from build123d import *

# Parameters (mm, degrees)
BOSS_EXTRUDE1_DEPTH      = 3
BOSS_EXTRUDE1_DEPTH_BACK = 1
CHAMFER1_SIZE            = 0.5


with BuildPart() as part:
    # Sketch2 → Boss-Extrude1 (new, two sides: drawn at the far end of the back side and taken through both)
    with BuildSketch(Plane(origin=(0, 0, 0), x_dir=(1, 0, 0), z_dir=(0, 1, 0)).offset(-BOSS_EXTRUDE1_DEPTH_BACK)):
        with BuildLine():
            Line((-9.425, 0.3), (-9.425, 0.925))
            Line((-9.425, 0.925), (-0.925, 0.925))
            Line((-0.925, 0.925), (-0.925, 9.425))
            Line((-0.925, 9.425), (0, 9.425))
            Line((0, 9.425), (0.925, 9.425))
            Line((0.925, 9.425), (0.925, 0.925))
            Line((0.925, 0.925), (9.425, 0.925))
            Line((9.425, 0.925), (9.425, 0.3))
            Line((9.425, 0.3), (11.446169588, 0.3))
            ThreePointArc((11.446169588, 0.3), (0, 11.45010036), (-11.446169588, 0.3))
            Line((-11.446169588, 0.3), (-9.425, 0.3))
        make_face()
    extrude(amount=BOSS_EXTRUDE1_DEPTH + BOSS_EXTRUDE1_DEPTH_BACK)

    # Chamfer1
    chamfer1_edges = [part.edges().sort_by_distance(p)[0] for p in [
        (-5.175, -1, -0.925),
        (-0.925, -1, -5.175),
        (0.925, 1, -0.925),
        (-0.925, 1, -0.925),
        (0.925, -1, -5.175),
        (-5.175, 3, -0.925),
        (-0.925, 3, -5.175),
        (0.925, 3, -5.175),
        (5.175, 3, -0.925),
        (5.175, -1, -0.925),
    ]]
    chamfer(chamfer1_edges, length=CHAMFER1_SIZE)


solid = part.part
Design review of the part built by this model. Coordinates are the model's own, in mm. A direction names the side the tool comes from. Coordinates: 2 decimals unless noted, no trailing zeros. Order: outer loops, then holes, each group sorted by start corner. A loop starts at its lowest first (then second) coordinate and runs counter-clockwise, first axis right, second up.
Item 1: The part is to be moulded in two halves that separate along X. For faces 1 (the cylindrical face through (0.248, 0.972, -11.447)), 2 (the flat face through (5, 1, -0.925)), 3 (the flat face through (-10, 1, -0.3)), say which applies: pulls with the +X half, pulls with the -X half, needs draft (parallel to the pull), parting line crosses it, or undercut.
Item 2: Take a section at A-A, the plane y = 1.1. Write out the cut boundary in (x, z) (3 decimals), then the cut area to 3 significant figures.
Item 3: Take a section at C-C, the plane x = 0. Write out the cut boundary in (y, z) (3 decimals).
Item 4: Take a section at B-B, the plane z = -4.75. Write out the cut boundary in (x, y) (3 decimals), then the cut area to 3 significant figures.
Item 5: Take a section at D-D, the plane z = -3.25. Write out the cut boundary in (x, y) (3 decimals).
Item 6: For line 1 (X direction, y = -0.6, z = -0.75) (3 decimals); line 2 (Z direction, x = 6.5, y = 1.8) (3 decimals); line 3 (Z direction, x = 0, y = -0.15) (3 decimals), list the stretches that pass through material, from the lowest coordinate up.
Item 7: For faces 4 (the flat face through (2, -1, -6)), 5 (the flat face through (-0.925, 1, -5)), list the 3-axis set-ups (+Z, -Z, +X, -X, +Y, -Y) from which the entire face can be reached by the end or side of a thin tool; tool diameter is ignored.
Item 8: For pin 1 Ø0.9 at (y, z) = (1, -1) entering from +X; pin 2 Ø0.6 at (y, z) = (1, -1) entering from -X; pin 3 Ø1.5 at (y, z) = (0.5, -7) entering from -X, all flat-tipped, find the tip position at first contact; note any pin that passes through.
The answers:
1. face 1: parting line crosses it
1. face 2: undercut
1. face 3: needs draft
2. outline: (-11.446, -0.3) arc R11.45 ccw to (11.446, -0.3) - (9.425, -0.3) - (9.425, -0.925) - (1.425, -0.925) - (0.925, -1.425) - (0.925, -9.425) - (-0.925, -9.425) - (-0.925, -1.425) - (-1.425, -0.925) - (-9.425, -0.925) - (-9.425, -0.3) - close
2. area: 171 mm2
3. outline: (-1, -11.45) - (3, -11.45) - (3, -9.425) - (-1, -9.425) - close
4. outline: (-10.418, -1) - (-1.425, -1) - (-0.925, -0.5) - (-0.925, 2.5) - (-1.425, 3) - (-10.418, 3) - close; (0.925, -0.5) - (1.425, -1) - (10.418, -1) - (10.418, 3) - (1.425, 3) - (0.925, 2.5) - close
4. area: 75.4 mm2
5. outline: (-10.979, -1) - (-1.425, -1) - (-0.925, -0.5) - (-0.925, 2.5) - (-1.425, 3) - (-10.979, 3) - close; (0.925, -0.5) - (1.425, -1) - (10.979, -1) - (10.979, 3) - (1.425, 3) - (0.925, 2.5) - close
6. line 1: x = -11.426 to -9.425, 9.425 to 11.426
6. line 2: z = -9.426 to -0.925
6. line 3: z = -11.45 to -9.425
7. face 4: +Z, -Z, +X, -X, -Y
7. face 5: +Z, +Y, -Y
8. pin 1: stops at x = 11.44
8. pin 2: stops at x = -11.43
8. pin 3: stops at x = -9.59
